from build123d import *

# Parameters (mm, degrees)
SKIZZE1_W                       = 160
SKIZZE1_H                       = 65
AUFSATZ_LINEAR_AUSTRAGEN1_DEPTH = 10
M5_GEWINDEBOHRUNG1_D            = 4.2
M5_GEWINDEBOHRUNG1_DEPTH        = 14
M5_GEWINDEBOHRUNG1_CSINK_D      = 5.05
M5_GEWINDEBOHRUNG1_CSINK_ANGLE  = 90
M5_GEWINDEBOHRUNG1_TIP          = 1.2618073
SCHNITT_LINEAR_AUSTRAGEN1_DEPTH = 87.926693254
FASE1_SIZE                      = 1


with BuildPart() as part:
    # Skizze1 → Aufsatz-Linear austragen1 (new body)
    with BuildSketch(Plane.XY):
        Rectangle(SKIZZE1_W, SKIZZE1_H)
    extrude(amount=AUFSATZ_LINEAR_AUSTRAGEN1_DEPTH)

    # M5 Gewindebohrung1
    with Locations(Plane.XY.offset(10)):
        with Locations((-72, 7.5), (-72, -22.5), (72, -22.5), (72, 7.5)):
            CounterSinkHole(M5_GEWINDEBOHRUNG1_D / 2, M5_GEWINDEBOHRUNG1_CSINK_D / 2, depth=M5_GEWINDEBOHRUNG1_DEPTH, counter_sink_angle=M5_GEWINDEBOHRUNG1_CSINK_ANGLE)
            with Locations((0, 0, -(M5_GEWINDEBOHRUNG1_DEPTH + M5_GEWINDEBOHRUNG1_TIP / 2))):  # 118° drill point
                Cone(0, M5_GEWINDEBOHRUNG1_D / 2, M5_GEWINDEBOHRUNG1_TIP, mode=Mode.SUBTRACT)

    # Skizze4 → Schnitt-Linear austragen1 (cut, through all)
    with BuildSketch(Plane.XY.offset(10)):
        with BuildLine():
            Line((27.75, 27.5), (27.75, 17.5))
            ThreePointArc((27.75, 17.5), (25, 14.75), (22.25, 17.5))
            Line((22.25, 17.5), (22.25, 27.5))
            ThreePointArc((22.25, 27.5), (25, 30.25), (27.75, 27.5))
        make_face()
        with BuildLine():
            Line((57.25, 17.5), (57.25, 27.5))
            ThreePointArc((57.25, 27.5), (60, 30.25), (62.75, 27.5))
            Line((62.75, 27.5), (62.75, 17.5))
            ThreePointArc((62.75, 17.5), (60, 14.75), (57.25, 17.5))
        make_face()
        with BuildLine():
            Line((-57.25, 17.5), (-57.25, 27.5))
            ThreePointArc((-57.25, 27.5), (-60, 30.25), (-62.75, 27.5))
            Line((-62.75, 27.5), (-62.75, 17.5))
            ThreePointArc((-62.75, 17.5), (-60, 14.75), (-57.25, 17.5))
        make_face()
    extrude(amount=-SCHNITT_LINEAR_AUSTRAGEN1_DEPTH, mode=Mode.SUBTRACT)

    # Fase1
    fase1_edges = [part.edges().sort_by_distance(p)[0] for p in [
        (80, 0, 10),
        (0, 32.5, 10),
        (-80, 0, 10),
        (0, -32.5, 10),
    ]]
    chamfer(fase1_edges, length=FASE1_SIZE)


solid = part.part
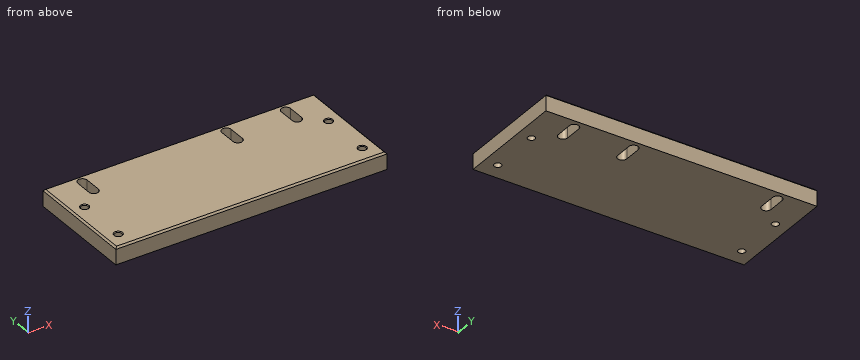
Input: part model. Units: mm. Frame: model coordinates. Give positions to 0.01 mm unless a question says otherwise; leave off trailing zeros. Order: outer loops, then holes, each group sorted by start corner. A loop starts at its lowest first (then second) coordinate and runs counter-clockwise, first axis right, second up. Notation, with made-up numbers: (84.25, -19) -> (110.25, -19) arc R20 ccw to (110.25, -7) -> close; hole circle Ø1 at (-12, -6.75). An arc over 180 degrees is marked (long way). Use one line per item in the form item = value.
1) Line query: probe 1 along X at (y, z) = (7.5, 7.5); probe 2 along X at (y, z) = (23, 5.25); probe 3 along Y at (x, z) = (-72, 3.75). Output: solid intervals per line, ascending.
Response values:
probe_1 = -80 to -74.1, -69.9 to 69.9, 74.1 to 80
probe_2 = -80 to -62.75, -57.25 to 22.25, 27.75 to 57.25, 62.75 to 80
probe_3 = -32.5 to -24.6, -20.4 to 5.4, 9.6 to 32.5
2) Section D-D, the plane y = 21.5. Return loops of the section in (x, z), and give its area (3 significant figures).
Response values:
outline = (-80, 0) -> (-62.75, 0) -> (-62.75, 10) -> (-79, 10) -> (-80, 9) -> close; (-57.25, 0) -> (22.25, 0) -> (22.25, 10) -> (-57.25, 10) -> close; (27.75, 0) -> (57.25, 0) -> (57.25, 10) -> (27.75, 10) -> close; (62.75, 0) -> (80, 0) -> (80, 9) -> (79, 10) -> (62.75, 10) -> close
area = 1,430 mm^2
3) Section A-A, the plane x = 25. Return loops of the section in (y, z), and give its area (3 significant figures).
Response values:
outline = (-32.5, 0) -> (14.75, 0) -> (14.75, 10) -> (-31.5, 10) -> (-32.5, 9) -> close; (30.25, 0) -> (32.5, 0) -> (32.5, 9) -> (31.5, 10) -> (30.25, 10) -> close
area = 494 mm^2
4) Section B-B, the plane y = 7.5. Return loops of the section in (x, z) (3 decimals).
Response values:
outline = (-80, 0) -> (-74.1, 0) -> (-74.1, 9.575) -> (-74.525, 10) -> (-79, 10) -> (-80, 9) -> close; (-69.9, 0) -> (69.9, 0) -> (69.9, 9.575) -> (69.475, 10) -> (-69.475, 10) -> (-69.9, 9.575) -> close; (74.1, 0) -> (80, 0) -> (80, 9) -> (79, 10) -> (74.525, 10) -> (74.1, 9.575) -> close
5) Section C-C, the plane x = 72. Return loops of the section in (y, z) (3 decimals), and give its area (3 significant figures).
Response values:
outline = (-32.5, 0) -> (-24.6, 0) -> (-24.6, 9.575) -> (-25.025, 10) -> (-31.5, 10) -> (-32.5, 9) -> close; (-20.4, 0) -> (5.4, 0) -> (5.4, 9.575) -> (4.975, 10) -> (-19.975, 10) -> (-20.4, 9.575) -> close; (9.6, 0) -> (32.5, 0) -> (32.5, 9) -> (31.5, 10) -> (10.025, 10) -> (9.6, 9.575) -> close
area = 565 mm^2
